```python
from build123d import *

# Parameters (mm, degrees)
SKETCH1_W                = 8
SKETCH1_H                = 7
BOSS_EXTRUDE1_DEPTH      = 192
SKETCH2_W                = 5
SKETCH2_H                = 3
CUT_EXTRUDE1_DEPTH       = 192
BOSS_EXTRUDE2_DEPTH      = 0.001
BOSS_EXTRUDE2_DEPTH_BACK = 3


with BuildPart() as part:
    # Sketch1 → Boss-Extrude1 (new body)
    with BuildSketch(Plane.XY):
        Rectangle(SKETCH1_W, SKETCH1_H)
    extrude(amount=BOSS_EXTRUDE1_DEPTH)

    # Sketch2 → Cut-Extrude1 (cut)
    with BuildSketch(Plane.XY.offset(192)):
        with Locations((-1.5, 0)):
            Rectangle(SKETCH2_W, SKETCH2_H)
    extrude(amount=-CUT_EXTRUDE1_DEPTH, mode=Mode.SUBTRACT)

    # Sketch3 → Boss-Extrude2 (add, two sides: drawn at the far end of the back side and taken through both)
    with BuildSketch(Plane(origin=(4, 0, 0), x_dir=(0, 0, -1), z_dir=(1, 0, 0)).offset(-BOSS_EXTRUDE2_DEPTH_BACK)):
        Polygon((0, -3.5), (-188.401251416, -40.121493492), (-188.401251416, -3.5), (-192, -3.5), (-192, 3.5), (0, 3.5), align=None)
    extrude(amount=BOSS_EXTRUDE2_DEPTH + BOSS_EXTRUDE2_DEPTH_BACK)


solid = part.part
```
The listing builds one solid part. Answer for the finished solid, in the listing's coordinates (mm). A direction names the side the tool comes from. Round coordinates to 2 decimals unless told otherwise and drop trailing zeros. Order: outer loops, then holes, each group sorted by start corner. A loop starts at its lowest first (then second) coordinate and runs counter-clockwise, first axis right, second up. Notation, with made-up numbers: (75.25, 18) -> (111.25, 18) arc R14 cw to (111.25, 28) -> close; hole circle Ø3 at (-25.75, 11.5). An arc over 180 degrees is marked (long way). Answer as CSV lines item,"result". Start each with the question number.
(1) A tool of negligible diameter and unlimited length cuts with its end or side. For faces 4 (the face through (1, -13, 135)), 5 (the face through (0, 3.5, 95)), 6 (the face through (-2, -1.5, 97)), from which of +Z, -Z, +X, -X, +Y, -Y can it reach the whole face along a straight path? Write none if from no direction.
(2) Flat-ended cylindrical pins translate along their axes: pin 1 Ø18.5 at (y, z) = (-30.5, 133) entering from -X; pin 2 Ø8 at (y, z) = (-13.5, 47) entering from +X; pin 3 Ø1.5 at (x, y) = (2.5, -20.5) entering from +Z; pin 4 Ø3 at (x, z) = (1, 116) entering from -Y. Find the tip coordinate at first contact, or state that the pin passes through.
(3) The part is cut by section D-D (z = 25.5). Determine the outline of the cut face in (x, y), then the cut area to 3 significant figures.
(4) For a pull along Y with two mould halves and no side action, classify faces 1 (the face through (1, 0, 97)), 2 (the face through (2, -22, 188.401)), 3 (the face through (2.479, -21.554, 92.882)) as +Y half, -Y half, draft (parallel to the pull), parting line (faces both ways), or undercut.
(5) The part is cut by section B-B (z = 153.5). Determine the outline of the cut face in (x, y), then the cut area to 3 significant figures.
(6) Find the intervals of material crossed by probe 1 along Y at (x, z) = (0, 97); probe 2 along X at (y, z) = (1, 84.5); probe 3 along Y at (x, z) = (2.75, 94), in increasing order. Write a range as from..to.
(7) The part is cut by section C-C (y = -20.5). Determine the outline of the cut face in (x, z).
(8) The part is cut by section A-A (x = -1.5). Determine the outline of the cut face in (y, z), then the cut area to 3 significant figures.
Evaluation:
1,face 4,"+Z, -Z, -X, -Y"
1,face 5,"+Z, -Z, +X, -X, +Y"
1,face 6,"+Z, -Z, -X"
2,pin 1,"x = 1"
2,pin 2,"x = 4"
2,pin 3,"z = 188.4"
2,pin 4,"y = -26.34"
3,outline,"(-4, -3.5) -> (1, -3.5) -> (1, -8.46) -> (4, -8.46) -> (4, 3.5) -> (-4, 3.5) -> (-4, 1.5) -> (1, 1.5) -> (1, -1.5) -> (-4, -1.5) -> close"
3,area,"55.9 mm²"
4,face 1,"undercut"
4,face 2,"draft"
4,face 3,"-Y half"
5,outline,"(-4, -3.5) -> (1, -3.5) -> (1, -33.34) -> (4, -33.34) -> (4, 3.5) -> (-4, 3.5) -> (-4, 1.5) -> (1, 1.5) -> (1, -1.5) -> (-4, -1.5) -> close"
5,area,"131 mm²"
6,probe 1,"-3.5..-1.5, 1.5..3.5"
6,probe 2,"1..4"
6,probe 3,"-21.77..3.5"
7,outline,"(1, 87.46) -> (4, 87.46) -> (4, 188.4) -> (1, 188.4) -> close"
8,outline,"(-3.5, 0) -> (-1.5, 0) -> (-1.5, 192) -> (-3.5, 192) -> close; (1.5, 0) -> (3.5, 0) -> (3.5, 192) -> (1.5, 192) -> close"
8,area,"768 mm²"
